Autodesk Inventor part; units mm, degrees
ref_plane "YZ Plane" through (0, 0, 0) normal (1, 0, 0) x (0, 1, 0)
ref_plane "XZ Plane" through (0, 0, 0) normal (0, 1, 0) x (-1, 0, 0)
ref_plane "XY Plane" through (0, 0, 0) normal (0, 0, 1) x (1, 0, 0)
ref_plane "Work Plane1" through (0, 0, 0) normal (0, 0, 1) x (1, 0, 0)
sketch "Sketch1" plane through (0, 0, 0) normal (0, 0, 1) x (1, 0, 0)
  line L0 (0, 0) -> (150, 0)
  line L1 (150, 0) -> (150, 6.35)
  line L2 (0, 6.35) -> (150, 6.35)
  line L3 (0, 0) -> (0, 6.35)
  line L4 (-41.185, 45.466) -> (-34.327, 45.466)
  line L5 (0, 6.35) -> (0, 45.466)
  line L6 (150, 6.35) -> (150, 45.466)
  line L7 (0, 45.466) -> (150, 45.466) construction
  line L8 (75, 45.466) -> (75, 96.266) construction
  line L9 (75, 96.266) -> (75, 248.666) construction
  line L10 (59.506, 80.772) -> (90.494, 80.772)
  line L11 (90.494, 80.772) -> (90.494, 111.76)
  line L12 (90.494, 111.76) -> (59.506, 111.76)
  line L13 (59.506, 111.76) -> (59.506, 80.772)
  line L14 (59.506, 80.772) -> (90.494, 111.76) construction
  line L15 (90.494, 80.772) -> (59.506, 111.76) construction
  line L16 (90.494, 118.11) -> (90.494, 105.41) construction
  line L17 (88.994, 118.11) -> (88.994, 105.41)
  line L18 (91.994, 105.41) -> (91.994, 118.11)
  arc A0 (91.994, 118.11) -> (88.994, 118.11) centre (90.494, 118.11) ccw
  arc A1 (88.994, 105.41) -> (91.994, 105.41) centre (90.494, 105.41) ccw
  line L19 (90.494, 74.422) -> (90.494, 87.122) construction
  line L20 (91.994, 74.422) -> (91.994, 87.122)
  line L21 (88.994, 87.122) -> (88.994, 74.422)
  arc A2 (88.994, 74.422) -> (91.994, 74.422) centre (90.494, 74.422) ccw
  arc A3 (91.994, 87.122) -> (88.994, 87.122) centre (90.494, 87.122) ccw
  line L22 (59.506, 105.41) -> (59.506, 118.11) construction
  line L23 (61.006, 105.41) -> (61.006, 118.11)
  line L24 (58.006, 118.11) -> (58.006, 105.41)
  arc A4 (58.006, 105.41) -> (61.006, 105.41) centre (59.506, 105.41) ccw
  arc A5 (61.006, 118.11) -> (58.006, 118.11) centre (59.506, 118.11) ccw
  line L25 (59.506, 74.422) -> (59.506, 87.122) construction
  line L26 (61.006, 74.422) -> (61.006, 87.122)
  line L27 (58.006, 87.122) -> (58.006, 74.422)
  arc A6 (58.006, 74.422) -> (61.006, 74.422) centre (59.506, 74.422) ccw
  arc A7 (61.006, 87.122) -> (58.006, 87.122) centre (59.506, 87.122) ccw
  line L28 (0, 45.466) -> (0, 248.666)
  line L29 (150, 45.466) -> (150, 248.666)
  circle A8 centre (75, 248.666) radius 75
  circle A9 centre (75, 316.966) radius 5.1943
  circle A10 centre (6.7, 248.666) radius 5.1943
  circle A11 centre (75, 180.366) radius 5.1943
  circle A12 centre (143.3, 248.666) radius 5.1943
  circle A13 centre (75, 248.666) radius 74.3
  circle A14 centre (75, 248.666) radius 62.3
  circle A15 centre (143.3, 248.666) radius 2.5
  circle A16 centre (75, 316.966) radius 2.5
  circle A17 centre (6.7, 248.666) radius 2.5
  circle A18 centre (75, 180.366) radius 2.5
  circle A19 centre (75, 96.266) radius 11.493 construction
  line L30 (75, 89.916) -> (75, 102.616) construction
  line L31 (63.507, 89.916) -> (63.507, 102.616)
  line L32 (86.493, 102.616) -> (86.493, 89.916)
  arc A20 (63.507, 89.916) -> (86.493, 89.916) centre (75, 89.916) ccw
  arc A21 (86.493, 102.616) -> (63.507, 102.616) centre (75, 102.616) ccw
  dimension "d0" = 50.8
  dimension "d1" = 152.4
  dimension "d2" = 30.988
  dimension "d3" = 30.988
  dimension "d4" = 6.35
  dimension "d5" = 3
  dimension "d6" = 6.35
  dimension "d7" = 3
  dimension "d8" = 6.35
  dimension "d9" = 3
  dimension "d10" = 6.35
  dimension "d11" = 3
  dimension "d14" = 5
  dimension "d17" = 360
  dimension "d19" = 6.35
extrude "Extrusion1" add sketch "Sketch1" along normal blind 6.35 contours L3 L2 L1 L0 | L5 L28 A8 L29 L6 L2 | A8 | L26 A7 L13 A4 L23 L12 A21 L31 A20 L10 | A20 L32 A21 L12 L17 A1 L11 A3 L21 L10 | A9 | A10 | A11 | A12 | A13
properties part number "SideBoard"
Check sheet for the modelled part. Datum: model origin and axes. Units: mm. A direction names the side the tool comes from. Coordinates: 2 decimals unless noted, no trailing zeros. Write each loop counter-clockwise with the first axis right and the second up, starting at its lowest first coordinate (ties: lowest second). Pieces come first, ordered by that corner, then holes. Notation, with made-up numbers: (32, 58) - (53, 58) arc R16 cw to (53, 89) - close; hole circle Ø3 at (-37, 34.25). An arc over 180 degrees is marked (long way). One line per question, with ' | ' between items.
Item 1: Sectioned sample at C-C on z = 4.5. Give the number of separate pieces and of enclosed holes in the cut face, plus the area to 3 significant figures.
Determined:
separate pieces: 1 | enclosed holes: 10 | area: 33,000 mm2
Item 2: Sectioned sample at B-B on x = 40. Record the boundary of the cut face in (y, z), plus the area to 3 significant figures.
Determined:
outline: (0, 0) - (197.13, 0) - (197.13, 6.35) - (0, 6.35) - close; (300.21, 0) - (315, 0) - (315, 6.35) - (300.21, 6.35) - close | area: 1,350 mm2
Item 3: Sectioned sample at A-A on y = 227.5. Record the boundary of the cut face in (x, z).
Determined:
outline: (0, 0) - (16.41, 0) - (16.41, 6.35) - (0, 6.35) - close; (133.59, 0) - (150, 0) - (150, 6.35) - (133.59, 6.35) - close
Item 4: Access from +Z, -Z, +X, -X, +Y, -Y to the whole of each face (thin tool, end or side, straight path). Record for faces 5 (the face through (74, 128, 6.35)), 6 (the face through (86.493, 96, 3)).
Determined:
face 5: +Z, +X, -X, +Y, -Y | face 6: +Z, -Z
Item 5: Gauge pin test, flat ends, axial feed: P1, Ø4.5, axis at x = 143.3, y = 248.666, coming from the -Z side; P2, Ø3, axis at y = 82.5, z = 3, coming from the -X side. Record the tip position at first contact, or that the pin passes through.
Determined:
P1: passes through | P2: stops at x = 0
Item 6: Thickness scan on line 1 (Y direction, x = 75, z = 5); line 2 (X direction, y = 107.5, z = 3.75); line 3 (Y direction, x = 65, z = 5.5). Record the ranges inside material, lowest first. Write a range as [from, to].
Determined:
line 1: y = [0, 78.42], [114.11, 177.87], [182.87, 186.37], [310.97, 314.47], [319.47, 323.67] | line 2: x = [0, 58.01], [61.01, 64.6], [85.4, 88.99], [91.99, 150] | line 3: y = [0, 84.25], [108.28, 187.17], [310.16, 323]
Item 7: Mould release check, pull along Y, two halves, no side actions. Record for faces 1 (the face through (74, 0, 3)), 2 (the face through (74, 128, 0)), 3 (the face through (73.351, 323.648, 3.131)), 4 (the face through (88.994, 112, 3)): pulls with the +Y half, pulls with the -Y half, needs draft (parallel to the pull), parting line crosses it, or undercut.
Determined:
face 1: pulls with the -Y half | face 2: needs draft | face 3: pulls with the +Y half | face 4: undercut
